from build123d import *

# Parameters (mm, degrees)
BOSS_EXTRUDE1_DEPTH = 30
SKETCH2_W           = 85.324686191
SKETCH2_H           = 2
BOSS_EXTRUDE2_DEPTH = 5


with BuildPart() as part:
    # Sketch1 → Boss-Extrude1 (new body)
    with BuildSketch(Plane.XY):
        Polygon((41.685097369, 7.4365364), (-43.314902631, 0), (11.685097369, 0), (11.685097369, 3), (41.685097369, 3), align=None)
    extrude(amount=BOSS_EXTRUDE1_DEPTH)

    # Sketch2 → Boss-Extrude2 (add)
    with BuildSketch(Plane(origin=(-0.32902535, 3.760776954, 0), x_dir=(0.9961946980917462, 0.08715574274765156, 0), z_dir=(-0.08715574274765156, 0.9961946980917462, 0))):
        with Locations((-0.487733254, -29)):
            Rectangle(SKETCH2_W, SKETCH2_H)
        with Locations((-0.487733254, -1)):
            Rectangle(SKETCH2_W, SKETCH2_H)
    extrude(amount=BOSS_EXTRUDE2_DEPTH)


solid = part.part
Geometry check sheet. Reference: the model listing, model coordinates, mm. A direction names the side the tool comes from. Give positions to 0.01 mm unless a question says otherwise; leave off trailing zeros. Write each loop counter-clockwise with the first axis right and the second up, starting at its lowest first coordinate (ties: lowest second). Pieces come first, ordered by that corner, then holes. Notation, with made-up numbers: M 61.5,18.5 L 86.5,18.5 A31 cw 86.5,56.5 Z; hole C 81,-30.75 d6. An arc over 180 degrees is marked long. Answer as CSV lines item,"result". Start each with the question number.
Q1. Section check B-B, the plane y = 8.5. Record the cut outline in (x, z), then the cut area to 3 significant figures.
Q2. Section check D-D, the plane y = 2. Record the cut outline in (x, z), then the cut area to 3 significant figures.
Q3. Material ranges on L1, parallel to Z at x = -8.5, y = 5.25; L2, parallel to Y at x = -38, z = 13 (3 decimals); L3, parallel to Y at x = 4.5, z = 27.25, recorded low to high.
Q4. Release check for a two-part mould opening along Z. For faces 4 (the face through (-43.53, 2.46, 1.01)), 5 (the face through (-0.22, 3.77, 14.82)), 6 (the face through (-2, 5, 0)), 7 (the face through (-2, 6, 28)) record: pulls with the +Z half, pulls with the -Z half, needs draft (parallel to the pull), parting line crosses it, or undercut.
Q5. Section check A-A, the plane z = 7.5. Record the cut outline in (x, y).
Q6. Tool access check on faces 1 (the face through (26, 3, 15)), 2 (the face through (41.47, 9.89, 1.01)), 3 (the face through (-2, 6, 2)). Record the directions out of +Z, -Z, +X, -X, +Y, -Y that give a thin tool (end or side, any length) a straight path to the whole face; none if there is none.
Q7. Section check C-C, the plane x = 15. Record the cut outline in (y, z), then the cut area to 3 significant figures.
Geometry says:
1,outline,"M -3.53,0 L 41.59,0 L 41.59,2 L -3.53,2 Z; M -3.53,28 L 41.59,28 L 41.59,30 L -3.53,30 Z"
1,area,"180 mm^2"
2,outline,"M -43.49,0 L 11.69,0 L 11.69,30 L -43.49,30 L -43.49,28 L -20.45,28 L -20.45,2 L -43.49,2 Z"
2,area,"1,060 mm^2"
3,L1,"0 to 2, 28 to 30"
3,L2,"0 to 0.465"
3,L3,"0 to 4.18"
4,face 4,"needs draft"
4,face 5,"undercut"
4,face 6,"pulls with the -Z half"
4,face 7,"undercut"
5,outline,"M -43.31,0 L 11.69,0 L 11.69,3 L 41.69,3 L 41.69,7.44 Z"
6,face 1,"+Z, -Z, +X, -Y"
6,face 2,"+Z, -Z, +X, +Y"
6,face 3,"-X, +Y"
7,outline,"M 3,0 L 10.12,0 L 10.12,2 L 5.1,2 L 5.1,28 L 10.12,28 L 10.12,30 L 3,30 Z"
7,area,"83.1 mm^2"
